```python
from build123d import *

# Parameters (mm, degrees)
ESQUISSE1_W             = 100.5
ESQUISSE1_H             = 100
BOSS_EXTRU_1_DEPTH      = 20
ESQUISSE2_W             = 9.5
ESQUISSE2_H             = 100
ENL_V_MAT_EXTRU_1_DEPTH = 17.1
ESQUISSE3_R             = 2.5
ENL_V_MAT_EXTRU_2_DEPTH = 16
ESQUISSE4_R             = 2.5
ENL_V_MAT_EXTRU_3_DEPTH = 16
ESQUISSE5_R             = 2.5
ENL_V_MAT_EXTRU_4_DEPTH = 21
ESQUISSE6_R             = 5
ENL_V_MAT_EXTRU_5_DEPTH = 21
ESQUISSE7_R             = 30
ENL_V_MAT_EXTRU_6_DEPTH = 4
ESQUISSE8_R             = 19
ENL_V_MAT_EXTRU_7_DEPTH = 4
ESQUISSE9_R             = 2.5
ENL_V_MAT_EXTRU_8_DEPTH = 13
ESQUISSE11_R            = 18
ENL_V_MAT_EXTRU_9_DEPTH = 21


with BuildPart() as part:
    # Esquisse1 → Boss.-Extru.1 (new body)
    with BuildSketch(Plane(origin=(0, 0, 0), x_dir=(1, 0, 0), z_dir=(0, 1, 0))):
        Rectangle(ESQUISSE1_W, ESQUISSE1_H)
    extrude(amount=BOSS_EXTRU_1_DEPTH)

    # Esquisse2 → Enlèv. mat.-Extru.1 (cut)
    with BuildSketch(Plane(origin=(0, 20, 0), x_dir=(1, 0, 0), z_dir=(0, 1, 0))):
        with Locations((45.5, 0)):
            Rectangle(ESQUISSE2_W, ESQUISSE2_H)
        with Locations((-45.5, 0)):
            Rectangle(ESQUISSE2_W, ESQUISSE2_H)
    extrude(amount=-ENL_V_MAT_EXTRU_1_DEPTH, mode=Mode.SUBTRACT)

    # Esquisse3 → Enlèv. mat.-Extru.2 (cut)
    with BuildSketch(Plane.ZY.offset(40.75)):
        with Locations((-40, 10.9)):
            Circle(ESQUISSE3_R)
        with Locations((-20, 10.9)):
            Circle(ESQUISSE3_R)
        with Locations((0, 10.9)):
            Circle(ESQUISSE3_R)
        with Locations((20, 10.9)):
            Circle(ESQUISSE3_R)
        with Locations((40, 10.9)):
            Circle(ESQUISSE3_R)
    extrude(amount=-ENL_V_MAT_EXTRU_2_DEPTH, mode=Mode.SUBTRACT)

    # Esquisse4 → Enlèv. mat.-Extru.3 (cut)
    with BuildSketch(Plane(origin=(40.75, 0, 0), x_dir=(0, 0, -1), z_dir=(1, 0, 0))):
        with Locations((-20, 10.9)):
            Circle(ESQUISSE4_R)
        with Locations((0, 10.9)):
            Circle(ESQUISSE4_R)
        with Locations((20, 10.9)):
            Circle(ESQUISSE4_R)
        with Locations((40, 10.9)):
            Circle(ESQUISSE4_R)
        with Locations((-40, 10.9)):
            Circle(ESQUISSE4_R)
    extrude(amount=-ENL_V_MAT_EXTRU_3_DEPTH, mode=Mode.SUBTRACT)

    # Esquisse5 → Enlèv. mat.-Extru.4 (cut, through all)
    with BuildSketch(Plane(origin=(0, 20, 0), x_dir=(1, 0, 0), z_dir=(0, 1, 0))):
        with Locations((0, -24.5)):
            Circle(ESQUISSE5_R)
        with Locations((-17.324116139, -17.324116139)):
            Circle(ESQUISSE5_R)
        with Locations((-24.5, 0)):
            Circle(ESQUISSE5_R)
        with Locations((-17.324116139, 17.324116139)):
            Circle(ESQUISSE5_R)
        with Locations((0, 24.5)):
            Circle(ESQUISSE5_R)
        with Locations((17.324116139, 17.324116139)):
            Circle(ESQUISSE5_R)
        with Locations((24.5, 0)):
            Circle(ESQUISSE5_R)
        with Locations((17.324116139, -17.324116139)):
            Circle(ESQUISSE5_R)
    extrude(amount=-ENL_V_MAT_EXTRU_4_DEPTH, mode=Mode.SUBTRACT)

    # Esquisse6 → Enlèv. mat.-Extru.5 (cut, through all)
    with BuildSketch(Plane(origin=(0, 20, 0), x_dir=(1, 0, 0), z_dir=(0, 1, 0))):
        Circle(ESQUISSE6_R)
    extrude(amount=-ENL_V_MAT_EXTRU_5_DEPTH, mode=Mode.SUBTRACT)

    # Esquisse7 → Enlèv. mat.-Extru.6 (cut)
    with BuildSketch(Plane.XZ):
        Circle(ESQUISSE7_R)
    extrude(amount=-ENL_V_MAT_EXTRU_6_DEPTH, mode=Mode.SUBTRACT)

    # Esquisse8 → Enlèv. mat.-Extru.7 (cut)
    with BuildSketch(Plane.XZ.offset(-4)):
        Circle(ESQUISSE8_R)
    extrude(amount=-ENL_V_MAT_EXTRU_7_DEPTH, mode=Mode.SUBTRACT)

    # Esquisse9 → Enlèv. mat.-Extru.8 (cut, through all)
    with BuildSketch(Plane.XZ.offset(-8)):
        with Locations((0, -12.5)):
            Circle(ESQUISSE9_R)
        with Locations((-10.825317547, -6.25)):
            Circle(ESQUISSE9_R)
        with Locations((-10.825317547, 6.25)):
            Circle(ESQUISSE9_R)
        with Locations((0, 12.5)):
            Circle(ESQUISSE9_R)
        with Locations((10.825317547, 6.25)):
            Circle(ESQUISSE9_R)
        with Locations((10.825317547, -6.25)):
            Circle(ESQUISSE9_R)
    extrude(amount=-ENL_V_MAT_EXTRU_8_DEPTH, mode=Mode.SUBTRACT)

    # Esquisse11 → Enlèv. mat.-Extru.9 (cut, through all)
    with BuildSketch(Plane(origin=(0, 20, 0), x_dir=(1, 0, 0), z_dir=(0, 1, 0))):
        with Locations((0, -50)):
            Circle(ESQUISSE11_R)
    extrude(amount=-ENL_V_MAT_EXTRU_9_DEPTH, mode=Mode.SUBTRACT)


solid = part.part
```
For this review, take the finished solid that the model builds, in its own axes (mm). A direction names the side the tool comes from. Coordinates: 2 decimals unless noted, no trailing zeros. Loops run counter-clockwise (first coordinate to the right, second up) from the corner with the lowest first, then second, coordinate; pieces in that order, holes last. Notation, with made-up numbers: (68.5, 22.25) -> (72.5, 22.25) arc R16 ccw to (72.5, 37.25) -> close; hole circle Ø4 at (10.5, 29). An arc over 180 degrees is marked (long way). Return JSON: item names as keys, results as strings. Group by question number.
(1) Mouldability with a two-part tool opening along Y and no side actions: class faces 5 (the flat face through (45, 2.9, -1)), 6 (the flat face through (-1, 10, -50)), 7 (the cylindrical face through (-32.862, 11.651, -37.615)), 8 (the cylindrical face through (32.9, 11, -17.5)) as pulls with the +Y half, pulls with the -Y half, needs draft (parallel to the pull), parting line crosses it, or undercut.
(2) To check wall thickness, follow L1, parallel to Z at x = 0, y = 15; L2, parallel to Z at x = 0, y = 5.7; L3, parallel to Y at x = 36, z = 0. State the ranges of each line that lie inside material, in increasing order.
(3) Consider section A-A, the plane x = 31.5. Give the boundary of the cut face in (y, z), plus the area to 3 significant figures.
(4) Consider section D-D, the plane z = 6.25. Give the boundary of the cut face in (x, y).
(5) Tool access review of faces 1 (the flat face through (-24.75, 11, 40)), 2 (the cylindrical face through (32.862, 11.651, -42.385)), 3 (the cylindrical face through (8.767, 5.972, -16.856)), 4 (the cylindrical face through (0, 10, 32)): name each direction out of +Z, -Z, +X, -X, +Y, -Y from which nothing blocks a thin tool from reaching the whole face with its end or side.
(6) Consider section B-B, the plane z = 36. Give the boundary of the cut face in (x, y).
(7) For pin 1 Ø5.5 at (y, z) = (10, 40) entering from -X; pin 2 Ø3 at (x, z) = (0, 12.5) entering from +Y; pin 3 Ø1.5 at (y, z) = (11, 19.5) entering from -X; pin 4 Ø3 at (y, z) = (4.5, 10.5) entering from +X, all flat-tipped, find the tip position at first contact; note any pin that passes through.
(8) Consider section C-C, the plane z = -40. Give the boundary of the cut face in (x, y).
Results below:
{
 "1": {"face 5": "pulls with the +Y half", "face 6": "needs draft", "face 7": "undercut", "face 8": "undercut"},
 "2": {"L1": "z = -50 to -27, -22 to -15, -10 to -5, 5 to 10, 15 to 22, 27 to 32", "L2": "z = -50 to -27, -22 to -19, 19 to 22, 27 to 32", "L3": "y = 0 to 8.4, 13.4 to 20"},
 "3": {"outline": "(0, -50) -> (20, -50) -> (20, 50) -> (0, 50) -> close; hole circle Ø5 at (10.9, -40); hole circle Ø5 at (10.9, -20); hole circle Ø5 at (10.9, 0); hole circle Ø5 at (10.9, 20); hole circle Ø5 at (10.9, 40)", "area": "1,900 mm2"},
 "4": {"outline": "(-50.25, 0) -> (-29.34, 0) -> (-29.34, 4) -> (-17.94, 4) -> (-17.94, 8) -> (-13.33, 8) -> (-13.33, 20) -> (-40.75, 20) -> (-40.75, 2.9) -> (-50.25, 2.9) -> close; (-8.33, 8) -> (8.33, 8) -> (8.33, 20) -> (-8.33, 20) -> close; (13.33, 8) -> (17.94, 8) -> (17.94, 4) -> (29.34, 4) -> (29.34, 0) -> (50.25, 0) -> (50.25, 2.9) -> (40.75, 2.9) -> (40.75, 20) -> (13.33, 20) -> close"},
 "5": {"face 1": "-X", "face 2": "+X", "face 3": "-Y", "face 4": "+Z, +Y, -Y"},
 "6": {"outline": "(-50.25, 0) -> (-11.31, 0) -> (-11.31, 20) -> (-40.75, 20) -> (-40.75, 2.9) -> (-50.25, 2.9) -> close; (11.31, 0) -> (50.25, 0) -> (50.25, 2.9) -> (40.75, 2.9) -> (40.75, 20) -> (11.31, 20) -> close"},
 "7": {"pin 1": "stops at x = -40.75", "pin 2": "passes through", "pin 3": "stops at x = -24.75", "pin 4": "stops at x = 40.75"},
 "8": {"outline": "(-50.25, 0) -> (50.25, 0) -> (50.25, 2.9) -> (40.75, 2.9) -> (40.75, 8.4) -> (24.75, 8.4) -> (24.75, 13.4) -> (40.75, 13.4) -> (40.75, 20) -> (-40.75, 20) -> (-40.75, 13.4) -> (-24.75, 13.4) -> (-24.75, 8.4) -> (-40.75, 8.4) -> (-40.75, 2.9) -> (-50.25, 2.9) -> close"}
}
